CAD build for the part. Positions are in the model's coordinates, mm. Face numbers are marked on the shaded views. Give positions to 0.01 mm unless a question says otherwise; leave off trailing zeros. Order: outer loops, then holes, each group sorted by start corner. A loop starts at its lowest first (then second) coordinate and runs counter-clockwise, first axis right, second up.
Item 1: Band-saw the part on B-B on y = 9.5. Give the cut face in (x, z).
Item 2: Band-saw the part on A-A on z = 4.2. Give the cut face in (x, y), plus the area to 3 significant figures.
Item 3: Wall check: L1, parallel to X at y = 0, z = 2.4; L2, parallel to Y at x = 11, z = 4.75. Give the ranges that are in metal, low to high.
Item 4: Flat gauge pins, fed straight in: P1, Ø1.5, axis at y = -12, z = 2.5, coming from the -X side; P2, Ø4.5, axis at x = 0, y = 46.5, coming from the +Z side; P3, Ø2, axis at y = 15, z = 0.5, coming from the -X side; P4, Ø3, axis at y = 23.5, z = 2, coming from the -X side. Where does each tip first touch, or does it go through?
Item 5: Band-saw the part on C-C on x = -14.5. Give the cut face in (y, z), plus the area to 3 significant figures.
Item 6: Two-plate mould, pull along Y, no slides. Class the marked faces 1, 2, 3 and 4: released by +Y, released by -Y, zero draft, split by the parting line, or undercut.
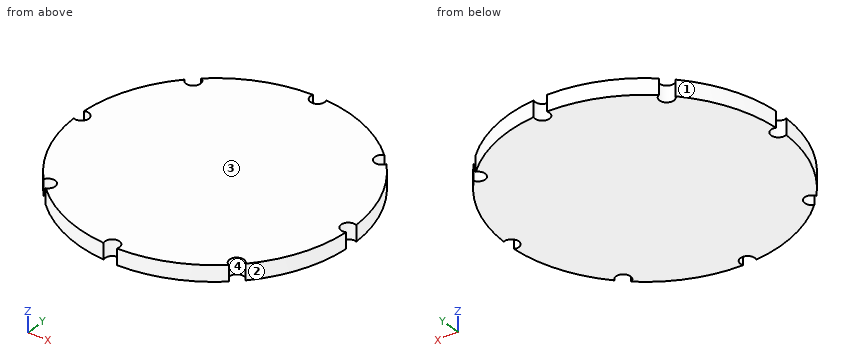
Autodesk Inventor part; units mm, degrees
ref_plane "YZ Plane" through (0, 0, 0) normal (1, 0, 0) x (0, 1, 0)
ref_plane "XZ Plane" through (0, 0, 0) normal (0, 1, 0) x (-1, 0, 0)
ref_plane "XY Plane" through (0, 0, 0) normal (0, 0, 1) x (1, 0, 0)
sketch "Sketch1" plane through (0, 0, 0) normal (0, 0, 1) x (1, 0, 0)
  circle A0 centre (0, 0) radius 47.5
  circle A1 centre (46.5, 0) radius 2.5
  dimension "d0" = 95
  dimension "d1" = 5
extrude "Extrusion1" add sketch "Sketch1" along normal blind 5.5 contours A0 A1 | A1 A0 picked at (46.4291, -0.6491) picked at (-16.8425, 0)
sketch "Sketch2" plane through (0, 0, 5.5) normal (0, 0, 1) x (1, 0, 0)
  circle A0 centre (46.5, 0) radius 2.5
  circle A1 centre (32.8805, 32.8805) radius 2.5
  circle A2 centre (0, 46.5) radius 2.5
  circle A3 centre (-32.8805, 32.8805) radius 2.5
  circle A4 centre (-46.5, 0) radius 2.5
  circle A5 centre (-32.8805, -32.8805) radius 2.5
  circle A6 centre (0, -46.5) radius 2.5
  circle A7 centre (32.8805, -32.8805) radius 2.5
  point P0 (0, 0)
  dimension "d4" = 5
  dimension "d7" = 360
extrude "Extrusion2" cut sketch "Sketch2" against normal blind 5.5
properties part number "tapa"
The answers:
1. outline: (-46.54, 0) - (46.54, 0) - (46.54, 5.5) - (-46.54, 5.5) - close
2. outline: (-47.44, -2.32) arc R47.5 ccw to (-35.18, -31.91) arc R2.5 cw (long way) to (-31.91, -35.18) arc R47.5 ccw to (-2.32, -47.44) arc R2.5 cw (long way) to (2.32, -47.44) arc R47.5 ccw to (31.91, -35.18) arc R2.5 cw (long way) to (35.18, -31.91) arc R47.5 ccw to (47.44, -2.32) arc R2.5 cw (long way) to (47.44, 2.32) arc R47.5 ccw to (35.18, 31.91) arc R2.5 cw (long way) to (31.91, 35.18) arc R47.5 ccw to (2.32, 47.44) arc R2.5 cw (long way) to (-2.32, 47.44) arc R47.5 ccw to (-31.91, 35.18) arc R2.5 cw (long way) to (-35.18, 31.91) arc R47.5 ccw to (-47.44, 2.32) arc R2.5 cw (long way) to start
2. area: 6,970 mm2
3. L1: x = -44 to 44
3. L2: y = -46.21 to 46.21
4. P1: stops at x = -46.15
4. P2: passes through
4. P3: stops at x = -45.39
4. P4: stops at x = -42.1
5. outline: (-45.23, 0) - (45.23, 0) - (45.23, 5.5) - (-45.23, 5.5) - close
5. area: 498 mm2
6. face 1: released by +Y
6. face 2: released by -Y
6. face 3: zero draft
6. face 4: undercut
